Part print with two shaded views. Sizes in mm from the minimum x, y, z corner. A direction names the side the tool comes from. Coordinates: 2 decimals unless noted, no trailing zeros. Loops run counter-clockwise (first coordinate to the right, second up) from the corner with the lowest first, then second, coordinate; pieces in that order, holes last. Notation, with made-up numbers: M 30,26.25 L 42,26.25 A31 ccw 42,65.25 Z; hole C -30,51.25 d11. An arc over 180 degrees is marked long. Use CSV: the item, a comma, the result in double quotes. Start each with the question number.
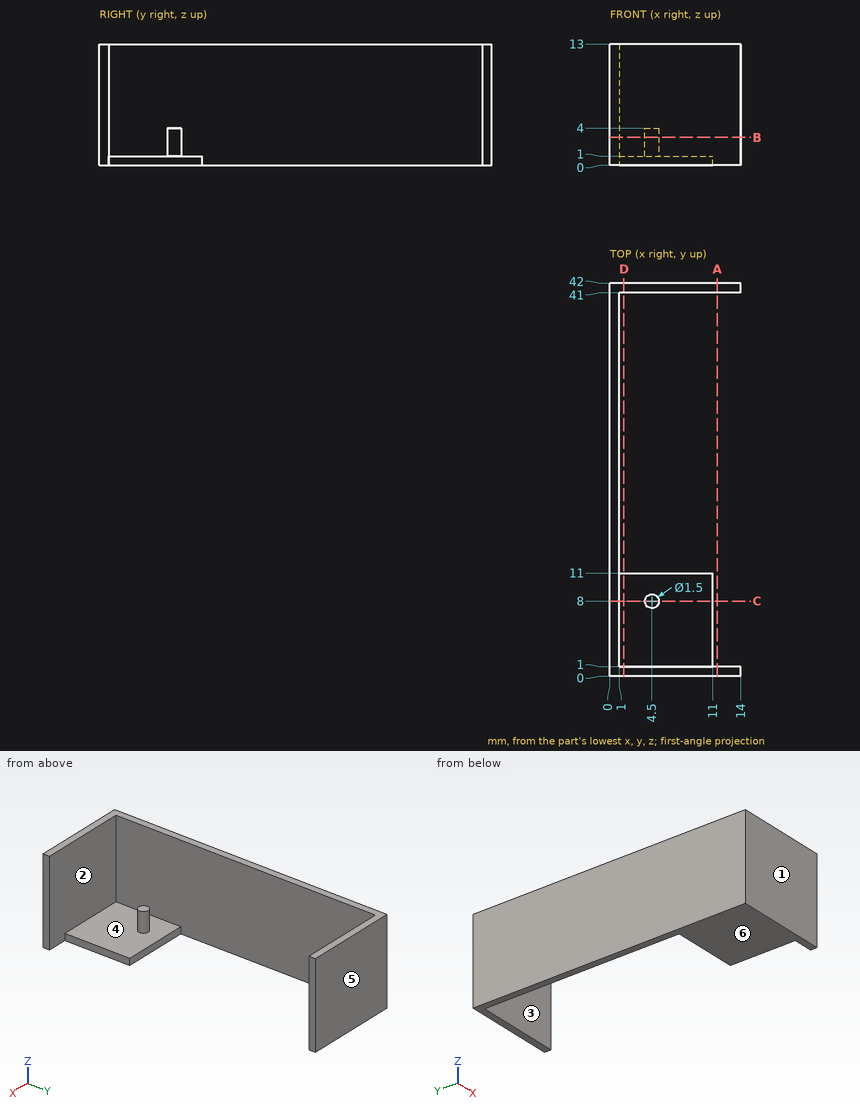
1. Slice it at D-D, the plane x = 1.5. List the corners of the cut face in (y, z).
2. Tool access for the marked faces 1, 2 and 3: list every direction of +Z, -Z, +X, -X, +Y, -Y with a clear straight run to the whole face (end or side of a thin tool).
3. Two-plate mould, pull along Y, no slides. Class the marked faces 4, 5 and 6: pulls with the +Y half, pulls with the -Y half, needs draft (parallel to the pull), parting line crosses it, or undercut.
4. Slice it at C-C, the plane y = 8. List the corners of the cut face in (x, z), and give its area (3 significant figures).
5. Slice it at B-B, the plane z = 3. List the corners of the cut face in (x, y).
6. Wall check: probe 1 along Y at (x, z) = (6.5, 2.75); probe 2 along X at (y, z) = (2, 9). Give the ranges that are in metal, low to high.
7. Pin check, flat tips, straight feed: pin 1 (6 mm diameter, centred on y = 34.5, z = 3, fed in from +X); pin 2 (0.8 mm diameter, centred on x = 4, y = 8, fed in from +Z); pin 3 (1 mm diameter, centred on y = 14.5, z = 8.5, fed in from -X); pin 4 (1 mm diameter, centred on x = 7, y = 5, fed in from +Z). Stop position of each tip, or through.
8. Slice it at A-A, the plane x = 11.5. List the corners of the cut face in (y, z).
Found:
1,outline,"M 0,0 L 11,0 L 11,1 L 1,1 L 1,13 L 0,13 Z; M 41,0 L 42,0 L 42,13 L 41,13 Z"
2,face 1,"+Z, -Z, +X, -X, -Y"
2,face 2,"+Z, +X"
2,face 3,"+Z, -Z, +X"
3,face 4,"undercut"
3,face 5,"pulls with the +Y half"
3,face 6,"needs draft"
4,outline,"M 0,0 L 11,0 L 11,1 L 5.25,1 L 5.25,4 L 3.75,4 L 3.75,1 L 1,1 L 1,13 L 0,13 Z"
4,area,"27.5 mm^2"
5,outline,"M 0,0 L 14,0 L 14,1 L 1,1 L 1,41 L 14,41 L 14,42 L 0,42 Z; C 4.5,8 d1.5"
6,probe 1,"0 to 1, 41 to 42"
6,probe 2,"0 to 1"
7,pin 1,"x = 1"
7,pin 2,"z = 4"
7,pin 3,"x = 0"
7,pin 4,"z = 1"
8,outline,"M 0,0 L 1,0 L 1,13 L 0,13 Z; M 41,0 L 42,0 L 42,13 L 41,13 Z"
